Check sheet for the modelled part. Datum: model origin and axes. Units: mm. A direction names the side the tool comes from. Coordinates: 2 decimals unless noted, no trailing zeros. Write each loop counter-clockwise with the first axis right and the second up, starting at its lowest first coordinate (ties: lowest second). Pieces come first, ordered by that corner, then holes. Notation, with made-up numbers: (75, 52) - (102, 52) arc R18 cw to (102, 77) - close; hole circle Ø10 at (76.5, 26.5). An arc over 180 degrees is marked (long way). Write each question's results on one line, items separated by ' | '.
from build123d import *

# Parameters (mm, degrees)
ESBO_O1_W                = 200
ESBO_O1_H                = 150
ESBO_O1_R                = 0.75
RESSALTO_EXTRUS_O1_DEPTH = 4
ESBO_O2_W                = 35
ESBO_O2_H                = 4
ESBO_O2_W_2              = 4
ESBO_O2_H_2              = 30
CORTE_EXTRUS_O1_DEPTH    = 5
ESBO_O3_W                = 200
ESBO_O3_H                = 15
CORTE_EXTRUS_O2_DEPTH    = 5
FURO_COM_FOLGA_DE_M41_D  = 4.5
ESBO_O5_R                = 3.4
CORTE_EXTRUS_O3_DEPTH    = 5


with BuildPart() as part:
    # Esboço1 → Ressalto-extrusão1 (new body)
    with BuildSketch(Plane(origin=(0, 0, 0), x_dir=(1, 0, 0), z_dir=(0, 1, 0))):
        Rectangle(ESBO_O1_W, ESBO_O1_H)
        with Locations((-37.8, 15.8)):
            Circle(ESBO_O1_R, mode=Mode.SUBTRACT)
        with Locations((37.8, 15.8)):
            Circle(ESBO_O1_R, mode=Mode.SUBTRACT)
        with Locations((37.8, -15.8)):
            Circle(ESBO_O1_R, mode=Mode.SUBTRACT)
        with Locations((-37.8, -15.8)):
            Circle(ESBO_O1_R, mode=Mode.SUBTRACT)
        Polygon((-35.65, -13.4), (35.65, -13.4), (35.65, -8), (38.15, -5.5), (38.15, 5.5), (35.65, 8), (35.65, 13.4), (-35.65, 13.4), align=None, mode=Mode.SUBTRACT)
    extrude(amount=RESSALTO_EXTRUS_O1_DEPTH)

    # Esboço2 → Corte-extrusão1 (cut, through all)
    with BuildSketch(Plane(origin=(0, 4, 0), x_dir=(1, 0, 0), z_dir=(0, 1, 0))):
        with Locations((-27.5, -73)):
            Rectangle(ESBO_O2_W, ESBO_O2_H)
        with Locations((27.5, -73)):
            Rectangle(ESBO_O2_W, ESBO_O2_H)
        with Locations((82.5, -73)):
            Rectangle(ESBO_O2_W, ESBO_O2_H)
        with Locations((-82.5, -73)):
            Rectangle(ESBO_O2_W, ESBO_O2_H)
        with Locations((98, 30)):
            Rectangle(ESBO_O2_W_2, ESBO_O2_H_2)
        with Locations((98, -30)):
            Rectangle(ESBO_O2_W_2, ESBO_O2_H_2)
        with Locations((-98, 30)):
            Rectangle(ESBO_O2_W_2, ESBO_O2_H_2)
        with Locations((-98, -30)):
            Rectangle(ESBO_O2_W_2, ESBO_O2_H_2)
    extrude(amount=-CORTE_EXTRUS_O1_DEPTH, mode=Mode.SUBTRACT)

    # Esboço3 → Corte-extrusão2 (cut, through all)
    with BuildSketch(Plane(origin=(0, 4, 0), x_dir=(1, 0, 0), z_dir=(0, 1, 0))):
        with Locations((0, 67.5)):
            Rectangle(ESBO_O3_W, ESBO_O3_H)
    extrude(amount=-CORTE_EXTRUS_O2_DEPTH, mode=Mode.SUBTRACT)

    # Furo com folga de M41 (through all)
    with Locations(Plane(origin=(-81, 4, -40), x_dir=(0, 0, 1), z_dir=(0, 1, 0))):
        with Locations((0, 0), (96, 0), (96, 162), (0, 162)):
            Hole(FURO_COM_FOLGA_DE_M41_D / 2)

    # Esboço5 → Corte-extrusão3 (cut, through all)
    with BuildSketch(Plane(origin=(0, 4, 0), x_dir=(1, 0, 0), z_dir=(0, 1, 0))):
        with Locations((-45, -41)):
            Circle(ESBO_O5_R)
        with Locations((0, -41)):
            Circle(ESBO_O5_R)
        with Locations((45, -41)):
            Circle(ESBO_O5_R)
    extrude(amount=-CORTE_EXTRUS_O3_DEPTH, mode=Mode.SUBTRACT)


solid = part.part
1. Sectioned sample at B-B (z = -40). Record the cut outline in (x, y).
Values follow:
outline: (-96, 0) - (-83.25, 0) - (-83.25, 4) - (-96, 4) - close; (-78.75, 0) - (78.75, 0) - (78.75, 4) - (-78.75, 4) - close; (83.25, 0) - (96, 0) - (96, 4) - (83.25, 4) - close
2. Material ranges on L1, parallel to X at y = 3.1, z = -40; L2, parallel to X at y = 1.1, z = -15.8; L3, parallel to X at y = 1.1, z = 41, recorded low to high. Write a range as [from, to].
Values follow:
L1: x = [-96, -83.25], [-78.75, 78.75], [83.25, 96] | L2: x = [-96, -38.55], [-37.05, 37.05], [38.55, 96] | L3: x = [-96, -48.4], [-41.6, -3.4], [3.4, 41.6], [48.4, 96]
3. Go/stop test with flat-tipped pins: pin 1 (2.5 mm diameter, centred on x = -81, z = -40, fed in from +Y); pin 2 (1.2 mm diameter, centred on y = 3, z = 73, fed in from +X); pin 3 (1.2 mm diameter, centred on x = -76, y = 2, fed in from +Z). Record where each tip stops, or that it passes through.
Values follow:
pin 1: passes through | pin 2: stops at x = 65 | pin 3: stops at z = 71
4. Sectioned sample at A-A (x = 0). Record the cut outline in (y, z).
Values follow:
outline: (0, -60) - (4, -60) - (4, -13.4) - (0, -13.4) - close; (0, 13.4) - (4, 13.4) - (4, 37.6) - (0, 37.6) - close; (0, 44.4) - (4, 44.4) - (4, 75) - (0, 75) - close
5. Access from +Z, -Z, +X, -X, +Y, -Y to the whole of each face (thin tool, end or side, straight path). Record for faces 1 (the flat face through (-65, 2, 73)), 2 (the flat face through (-45, 2, 73)), 3 (the flat face through (98, 2, -45)), 4 (the flat face through (35.65, 2, 11)).
Values follow:
face 1: +Z, -X, +Y, -Y | face 2: +Z, +Y, -Y | face 3: +X, +Y, -Y | face 4: +Y, -Y
6. Sectioned sample at C-C (z = 3.5). Record the cut outline in (x, y), then the cut area to 3 significant figures.
Values follow:
outline: (-100, 0) - (-35.65, 0) - (-35.65, 4) - (-100, 4) - close; (38.15, 0) - (100, 0) - (100, 4) - (38.15, 4) - close | area: 505 mm^2
7. Draft check along Z on faces 5 (the flat face through (-28, 2, 71)), 6 (the flat face through (-96, 2, 30)), 7 (the flat face through (-1, 4, 22)). Enter one of: pulls with the +Z half, pulls with the -Z half, needs draft (parallel to the pull), parting line crosses it, or undercut.
Values follow:
face 5: pulls with the +Z half | face 6: undercut | face 7: needs draft
8. Sectioned sample at D-D (x = -24). Record the cut outline in (y, z).
Values follow:
outline: (0, -60) - (4, -60) - (4, -13.4) - (0, -13.4) - close; (0, 13.4) - (4, 13.4) - (4, 71) - (0, 71) - close
